Design review of the part shown in the three views and the two pictorial views. Dimensions are in mm from the part's minimum x, y and z. A direction names the side the tool comes from. Give positions to 0.01 mm unless a question says otherwise; leave off trailing zeros. Loops run counter-clockwise (first coordinate to the right, second up) from the corner with the lowest first, then second, coordinate; pieces in that order, holes last. Notation, with made-up numbers: M -21,-22 L 22,-22 A22 ccw 22,2 Z; hole C -17.75,30.5 d1. An arc over 180 degrees is marked long. Return JSON: item names as keys, results as strings. Group by question number.
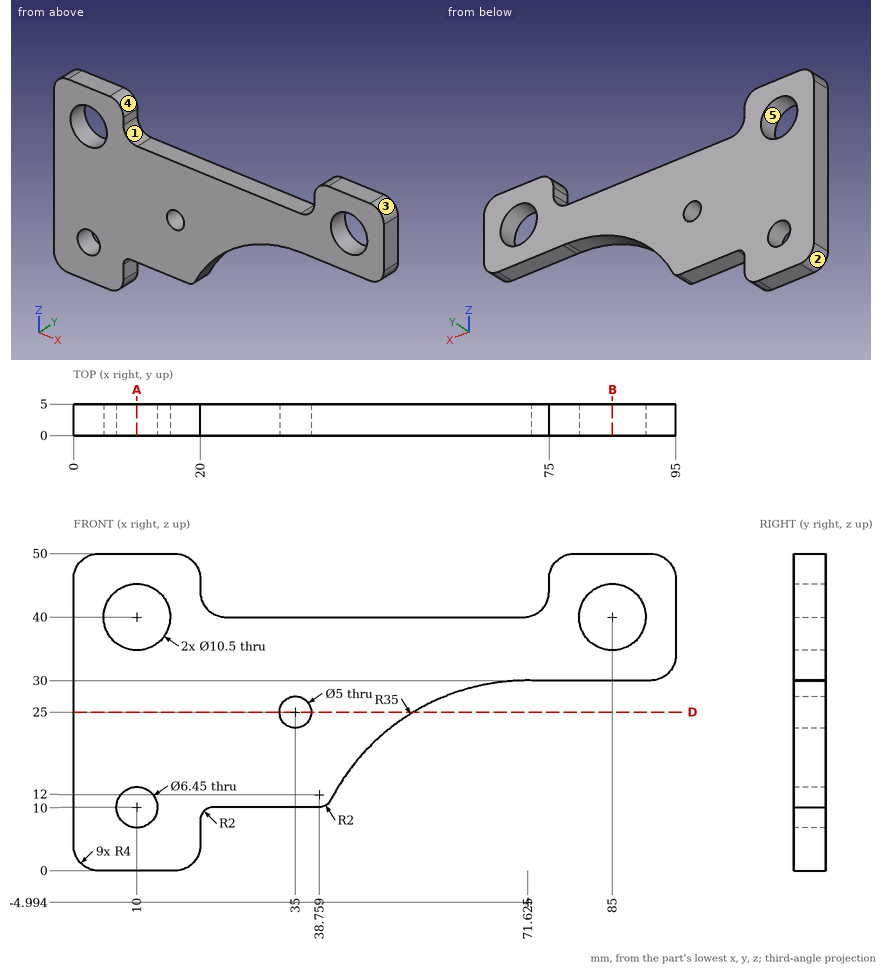
(1) For the marked faces 4 and 5, list the 3-axis set-ups (+Z, -Z, +X, -X, +Y, -Y) from which the entire face can be reached by the end or side of a thin tool; tool diameter is ignored.
(2) Mouldability with a two-part tool opening along X and no side actions: class the marked faces 1, 2 and 3 as released by +X, released by -X, zero draft, split by the parting line, or undercut.
(3) Add section D-D (z = 25). Write out the cut boundary in (x, y).
(4) For pin 1 (1.2 mm diameter, centred on y = 2.5, z = 6.5, fed in from +X); pin 2 (12 mm diameter, centred on x = 85, z = 40, fed in from +Y); pin 3 (2 mm diameter, centred on x = 38.5, y = 1, fed in from +Z); pin 4 (1.5 mm diameter, centred on x = 32, y = 3, fed in from -Z), all flat-tipped, find the tip position at first contact; note any pin that passes through.
(5) Add section B-B (x = 85). Write out the cut boundary in (y, z).
(6) For probe 1 along X at (y, z) = (2.65, 37); probe 2 along X at (y, z) = (4.05, 25) (1 decimal); probe 3 along Z at (x, y) = (37, 1.7), list the stretches that pass through material, from the lowest coordinate up.
(7) Add section A-A (x = 10). Count the separate pieces of the cut face and the enclosed holes in it, and give its area (3 significant figures).
Verdict:
{
 "1": {"face 4": "+Z, +Y, -Y", "face 5": "+Y, -Y"},
 "2": {"face 1": "undercut", "face 2": "released by -X", "face 3": "released by +X"},
 "3": {"outline": "M 0,0 L 32.5,0 L 32.5,5 L 0,5 Z; M 37.5,0 L 53.59,0 L 53.59,5 L 37.5,5 Z"},
 "4": {"pin 1": "stops at x = 20", "pin 2": "stops at y = 5", "pin 3": "stops at z = 40", "pin 4": "stops at z = 10"},
 "5": {"outline": "M 0,30 L 5,30 L 5,34.75 L 0,34.75 Z; M 0,45.25 L 5,45.25 L 5,50 L 0,50 Z"},
 "6": {"probe 1": "x = 0 to 5.69, 14.31 to 80.69, 89.31 to 95", "probe 2": "x = 0 to 32.5, 37.5 to 53.6", "probe 3": "z = 10 to 23.5, 26.5 to 40"},
 "7": {"separate pieces": "3", "enclosed holes": "0", "area": "165 mm²"}
}
